from build123d import *

# Parameters (mm, degrees)
SKETCH1_W           = 33
SKETCH1_H           = 33
BOSS_EXTRUDE1_DEPTH = 30
SKETCH2_R           = 16
CUT_EXTRUDE1_DEPTH  = 3
SKETCH3_R           = 1
CUT_EXTRUDE2_DEPTH  = 2
FILLET1_R           = 1


with BuildPart() as part:
    # Sketch1 → Boss-Extrude1 (new body)
    with BuildSketch(Plane(origin=(0, 0, 0), x_dir=(1, 0, 0), z_dir=(0, 1, 0))):
        Rectangle(SKETCH1_W, SKETCH1_H)
    extrude(amount=BOSS_EXTRUDE1_DEPTH)

    # Sketch2 → Cut-Extrude1 (cut)
    with BuildSketch(Plane(origin=(0, 30, 0), x_dir=(1, 0, 0), z_dir=(0, 1, 0))):
        Circle(SKETCH2_R)
    extrude(amount=-CUT_EXTRUDE1_DEPTH, mode=Mode.SUBTRACT)

    # Sketch3 → Cut-Extrude2 (cut)
    with BuildSketch(Plane.XZ):
        Circle(SKETCH3_R)
    extrude(amount=-CUT_EXTRUDE2_DEPTH, mode=Mode.SUBTRACT)

    # Fillet1
    fillet1_edges = [part.edges().sort_by_distance(p)[0] for p in [
        (-1, 2, 0),
    ]]
    fillet(fillet1_edges, radius=FILLET1_R)


solid = part.part
Read the model definition and answer for the solid it produces. Units are mm, in the model's axes. A direction names the side the tool comes from. Coordinates: 2 decimals unless noted, no trailing zeros. Loops run counter-clockwise (first coordinate to the right, second up) from the corner with the lowest first, then second, coordinate; pieces in that order, holes last. Notation, with made-up numbers: (45.25, 80) - (62.25, 80) arc R30 cw to (62.25, 113) - close; hole circle Ø7 at (-9.5, 35.25). An arc over 180 degrees is marked (long way). Answer in a Markdown table with one row per item.
Q1. Given P1, Ø1.5, axis at x = 0, z = 8, coming from the +Y side, flat-ended and moving along its own axis, determine where the tip first touches the part or whether it passes through.
Here are the results:
| item | result |
|---|---|
| P1 | stops at y = 27 |
Q2. Find section B-B on z = 0. Write down the section's boundary in (x, y), plus the area to 3 significant figures.
Here are the results:
| item | result |
|---|---|
| outline | (-16.5, 0) - (-1, 0) - (-1, 1) arc R1 cw to (1, 1) - (1, 0) - (16.5, 0) - (16.5, 30) - (16, 30) - (16, 27) - (-16, 27) - (-16, 30) - (-16.5, 30) - close |
| area | 890 mm^2 |
Q3. Find section D-D on x = 12. Write down the section's boundary in (y, z).
Here are the results:
| item | result |
|---|---|
| outline | (0, -16.5) - (30, -16.5) - (30, -10.58) - (27, -10.58) - (27, 10.58) - (30, 10.58) - (30, 16.5) - (0, 16.5) - close |
Q4. For faces 1 (the cylindrical face through (-0.217, 0.493, -0.976)), 2 (the flat face through (0, 15, -16.5)), determine the directions among +Z, -Z, +X, -X, +Y, -Y from which every point of the face is accessible in a straight line to the end or side of a thin tool.
Here are the results:
| item | result |
|---|---|
| face 1 | -Y |
| face 2 | -Z, +X, -X, +Y, -Y |
Q5. Straight lines are drawn through the part: line 1 along Z through (x, y) = (0, 0.65); line 2 along Z through (x, y) = (0, 28.65). For each, find the intervals that lie inside material, in ascending order. Write a range as [from, to].
Here are the results:
| item | result |
|---|---|
| line 1 | z = [-16.5, -1], [1, 16.5] |
| line 2 | z = [-16.5, -16], [16, 16.5] |
Q6. Find section A-A on x = 0. Write down the section's boundary in (y, z).
Here are the results:
| item | result |
|---|---|
| outline | (0, -16.5) - (30, -16.5) - (30, -16) - (27, -16) - (27, 16) - (30, 16) - (30, 16.5) - (0, 16.5) - (0, 1) - (1, 1) arc R1 cw to (1, -1) - (0, -1) - close |
Q7. The mould has two halves that part along Z. Classify faces 3 (the flat face through (0, 0, -4)), 4 (the flat face through (0, 27, 0)), 5 (the flat face through (0, 15, 16.5)), 6 (the cylindrical face through (-3.47, 28.52, 15.62)): pulls with the +Z half, pulls with the -Z half, needs draft (parallel to the pull), parting line crosses it, or undercut.
Here are the results:
| item | result |
|---|---|
| face 3 | needs draft |
| face 4 | undercut |
| face 5 | pulls with the +Z half |
| face 6 | undercut |
Q8. Find section C-C on z = 8.5. Write down the section's boundary in (x, y), plus the area to 3 significant figures.
Here are the results:
| item | result |
|---|---|
| outline | (-16.5, 0) - (16.5, 0) - (16.5, 30) - (13.56, 30) - (13.56, 27) - (-13.56, 27) - (-13.56, 30) - (-16.5, 30) - close |
| area | 909 mm^2 |
